Can you work these out from the model? Positions are in its coordinate system, mm. Face numbers are marked on the shaded views. A direction names the side the tool comes from. Coordinates: 2 decimals unless noted, no trailing zeros. Order: outer loops, then holes, each group sorted by start corner. A loop starts at its lowest first (then second) coordinate and runs counter-clockwise, first axis right, second up. Notation, with made-up numbers: (56, 77) -> (75, 77) arc R24 ccw to (75, 96) -> close; hole circle Ø9 at (5.5, 41). An arc over 180 degrees is marked (long way). Answer as a JSON object with one key per item and string values. Group by question number.
(1) I want a section at C-C, the plane z = -73.5. List the corners of the cut face in (x, y) for me.
(2) I want a section at B-B, the plane x = 16. List the corners of the cut face in (y, z) for me.
(3) Which directions (+Z, -Z, +X, -X, +Y, -Y) give clear straight access to the entire face, cutting with the end or side of a thin tool? Please do the marked faces 1 and 2.
(4) For pin 1 (6 mm diameter, centred on y = 13, z = -70.5, fed in from -X); pin 2 (5.5 mm diameter, centred on x = 16, y = 0, fed in from +Z); pin 3 (8 mm diameter, centred on y = -14, z = -67, fed in from +X), each with a flat end and sliding along its axis, tell me the tip position at first contact or that it passes through.
(5) I want a section at A-A, the plane y = 0. List the corners of the cut face in (x, z) for me.
(6) I want a section at D-D, the plane x = -5.5. List the corners of the cut face in (y, z) for me, plus the area to 3 significant figures.
(7) I need wall thicknesses on line 1 (Y direction, x = -16, z = -56); line 2 (Z direction, x = -14.5, y = 6.5); line 3 (X direction, y = -1, z = -4). Which ranges of each line are inside material? Lowest first, please.
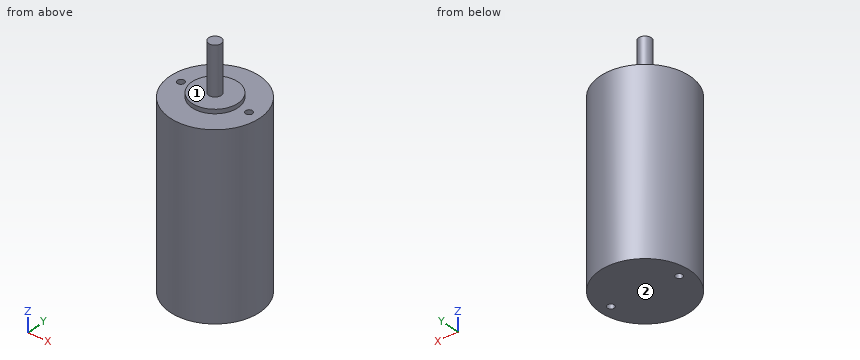
from build123d import *

# Parameters (mm, degrees)
F0_R     = 21.5
F1_DEPTH = 86
F2_R     = 11
F3_DEPTH = 2
F4_R     = 3
F5_DEPTH = 23
F7_D     = 3.3


with BuildPart() as f1:
    # F0 (on Top) → F1 (new body)
    with BuildSketch(Plane.XY):
        Circle(F0_R)
    extrude(amount=-F1_DEPTH)

    # F2 (on face) → F3 (join)
    with BuildSketch(Plane.XY):
        Circle(F2_R)
    extrude(amount=F3_DEPTH)

    # F4 (on face) → F5 (join)
    with BuildSketch(Plane.XY.offset(2)):
        Circle(F4_R)
    extrude(amount=F5_DEPTH)

    # F7 (through all)
    with Locations(Plane.XY):
        with Locations((-16, 0), (16, 0)):
            Hole(F7_D / 2)


solid = f1.part
Computed values:
{
 "1": {"outline": "circle Ø43 at (0, 0); hole circle Ø3.3 at (-16, 0); hole circle Ø3.3 at (16, 0)"},
 "2": {"outline": "(-14.36, -86) -> (-1.65, -86) -> (-1.65, 0) -> (-14.36, 0) -> close; (1.65, -86) -> (14.36, -86) -> (14.36, 0) -> (1.65, 0) -> close"},
 "3": {"face 1": "+Z", "face 2": "-Z, +X, -X, +Y, -Y"},
 "4": {"pin 1": "stops at x = -19.03", "pin 2": "stops at z = 0", "pin 3": "stops at x = 19.03"},
 "5": {"outline": "(-21.5, -86) -> (-17.65, -86) -> (-17.65, 0) -> (-21.5, 0) -> close; (-14.35, -86) -> (14.35, -86) -> (14.35, 0) -> (11, 0) -> (11, 2) -> (3, 2) -> (3, 25) -> (-3, 25) -> (-3, 2) -> (-11, 2) -> (-11, 0) -> (-14.35, 0) -> close; (17.65, -86) -> (21.5, -86) -> (21.5, 0) -> (17.65, 0) -> close"},
 "6": {"outline": "(-20.78, -86) -> (20.78, -86) -> (20.78, 0) -> (9.53, 0) -> (9.53, 2) -> (-9.53, 2) -> (-9.53, 0) -> (-20.78, 0) -> close", "area": "3,610 mm2"},
 "7": {"line 1": "y = -14.36 to -1.65, 1.65 to 14.36", "line 2": "z = -86 to 0", "line 3": "x = -21.48 to -17.31, -14.69 to 14.69, 17.31 to 21.48"}
}
